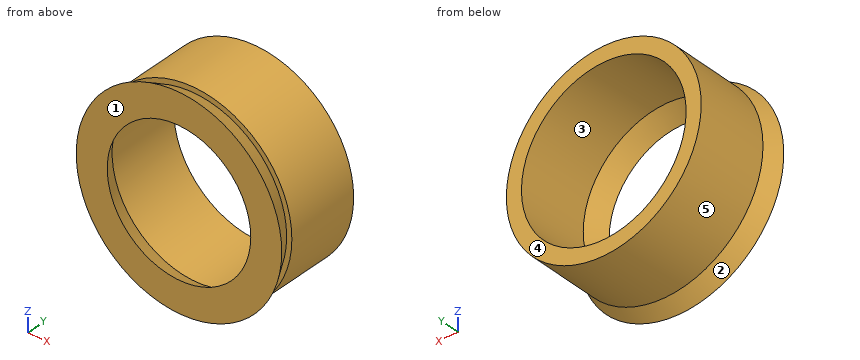
```python
from build123d import *

# Parameters (mm, degrees)
F0_R     = 532.5
F1_DEPTH = 400
F2_R     = 450
F3_DEPTH = 400
F4_R     = 504
F4_R_2   = 450
F5_DEPTH = 100
F5_TAPER = -30


with BuildPart() as f1:
    # F0 (on Front) → F1 (new body)
    with BuildSketch(Plane.XZ):
        Circle(F0_R)
    extrude(amount=F1_DEPTH)

    # F2 (on face) → F3 (cut)
    with BuildSketch(Plane.XZ.offset(400)):
        Circle(F2_R)
    extrude(amount=-F3_DEPTH, mode=Mode.SUBTRACT)

    # F4 (on face) → F5 (join)
    with BuildSketch(Plane.XZ.offset(400)):
        Circle(F4_R)
        Circle(F4_R_2, mode=Mode.SUBTRACT)
    extrude(amount=F5_DEPTH, taper=F5_TAPER)


solid = f1.part
```
Part model, mm, in its own coordinate system. Face numbers are marked on the shaded views. A direction names the side the tool comes from. Give positions to 0.01 mm unless a question says otherwise; leave off trailing zeros. Order: outer loops, then holes, each group sorted by start corner. A loop starts at its lowest first (then second) coordinate and runs counter-clockwise, first axis right, second up. Notation, with made-up numbers: M -7.5,6 L 12.5,6 A20 ccw 12.5,29 Z; hole C -11.5,84 d5. An arc over 180 degrees is marked long. Use a Markdown table: item, result. Add a question column.
(1) Probe line 1 along Z through (x, y) = (0, -260); line 2 along Z through (x, y) = (-13, -195); line 3 along Y through (x, z) = (-301, -422.5). List the from-to ranges inside material, lowest first. Write a range as [from, to].
(2) 3-axis set-ups, long thin cutter, end or side, ignore diameter. For the marked faces 1 and 2: which of +Z, -Z, +X, -X, +Y, -Y reach the whole face in a straight line?
(3) Saw through at A-A, the plane x = 0. Give the cut face in (y, z).
(4) Saw through at B-B, the plane y = -101. Give the cut face in (x, z), and give its area (3 significant figures).
(5) Mould opens along X. For the marked faces 3, 4 and 5 say: +X half, -X half, draft (parallel to the pull), parting line (faces both ways), or undercut.
(6) Drop flat-ended pins along their axis: P1, Ø1, axis at x = 181, y = -299, coming from the +Z side; P2, Ø8, axis at x = -284.5, y = -341, coming from the +Z side; P3, Ø10, axis at x = -268.5, y = -224, coming from the -Z side. Give the stop position or say it passes through.
Answer key:
| question | item | result |
|---|---|---|
| 1 | line 1 | [-532.5, -450], [450, 532.5] |
| 1 | line 2 | [-532.34, -449.81], [449.81, 532.34] |
| 1 | line 3 | [-500, -425.56], [-400, 0] |
| 2 | face 1 | +Z, -Z, +X, -X, -Y |
| 2 | face 2 | none |
| 3 | outline | M -500,-561.74 L -400,-504 L -400,-532.5 L 0,-532.5 L 0,-450 L -400,-450 L -500,-392.26 Z; M -500,392.26 L -400,450 L 0,450 L 0,532.5 L -400,532.5 L -400,504 L -500,561.74 Z |
| 4 | outline | C 0,0 d1065; hole C 0,0 d900 |
| 4 | area | 255,000 mm^2 |
| 5 | face 3 | undercut |
| 5 | face 4 | draft |
| 5 | face 5 | parting line |
| 6 | P1 | z = 500.98 |
| 6 | P2 | z = 452.63 |
| 6 | P3 | z = -462.74 |
